The listing builds one solid part. Answer for the finished solid, in the listing's coordinates (mm). A direction names the side the tool comes from. Round coordinates to 2 decimals unless told otherwise and drop trailing zeros. Loops run counter-clockwise (first coordinate to the right, second up) from the corner with the lowest first, then second, coordinate; pieces in that order, holes last. Notation, with made-up numbers: (81.5, -17.75) - (126.5, -17.75) arc R31 ccw to (126.5, 18.25) - close; hole circle Ø6 at (-29, 69.25). An arc over 180 degrees is marked (long way). One line per item, written item: value.
```python
from build123d import *

# Parameters (mm, degrees)
F2_DEPTH = 38.1
F3_DEPTH = 25.4


with BuildPart() as f2:
    # F0 (on Right) → F2 (new body)
    with BuildSketch(Plane.YZ):
        Polygon((0, 6.35), (0, 0), (25.4, 0), (25.4, 19.05), (19.05, 19.05), (19.05, 6.35), align=None)
    extrude(amount=F2_DEPTH)

    # F1 (on Front) → F3 (join)
    with BuildSketch(Plane.XZ):
        Polygon((0, 25.4), (0, 0), (38.1, 0), (38.1, 6.35), (12.7, 6.35), (12.7, 19.05), (12.7, 25.4), align=None)
    extrude(amount=-F3_DEPTH)


solid = f2.part
```
1) Each of these flat-tipped pins is pushed along its axis until it touches: pin 1 Ø7 at (x, y) = (30.5, 21) entering from +Z; pin 2 Ø5.5 at (y, z) = (11.5, 20) entering from +X; pin 3 Ø6.5 at (x, z) = (19.5, 14.5) entering from -Y. Where does it stop, or does it pass through?
Final values:
pin 1: z = 19.05
pin 2: x = 12.7
pin 3: y = 19.05
2) For faces 1 (the flat face through (25, 19.05, 13)), 2 (the flat face through (25, 22, 19.05)), 3 (the flat face through (19, 13, 0)), determine the directions among +Z, -Z, +X, -X, +Y, -Y from which every point of the face is accessible in a straight line to the end or side of a thin tool.
Final values:
face 1: +Z, +X, -Y
face 2: +Z, +X, +Y, -Y
face 3: -Z, +X, -X, +Y, -Y
3) Consider L1, parallel to Y at x = 34.5, z = 6.5; L2, parallel to Z at x = 20.5, y = 19.5; L3, parallel to X at y = 14.25, z = 9. Determine where each line is inside the solid, lowest interval first.
Final values:
L1: 19.05 to 25.4
L2: 0 to 19.05
L3: 0 to 12.7
4) A cutting plane is placed at B-B on x = 16.5. Give the vertices of the cut face in (y, z).
Final values:
outline: (0, 0) - (25.4, 0) - (25.4, 19.05) - (19.05, 19.05) - (19.05, 6.35) - (0, 6.35) - close
5) A cutting plane is placed at A-A on y = 23. Give the vertices of the cut face in (x, z), and give its area (3 significant figures).
Final values:
outline: (0, 0) - (38.1, 0) - (38.1, 19.05) - (12.7, 19.05) - (12.7, 25.4) - (0, 25.4) - close
area: 806 mm2
